```python
from build123d import *


with BuildPart() as part:
    # Esquisse1 → Révolution1 (revolve)
    with BuildSketch(Plane(origin=(0, 0, 0), x_dir=(0, 0, -1), z_dir=(1, 0, 0)), mode=Mode.PRIVATE) as r_volution1_sk:
        with BuildLine():
            Line((0, 1.5), (4, 1.5))
            Line((4, 1.5), (4, 2.15))
            Line((4, 2.15), (3, 2.15))
            ThreePointArc((3, 2.15), (3.6, 2.75), (3, 3.35))
            Line((3, 3.35), (4, 3.35))
            Line((4, 3.35), (4, 4))
            Line((4, 4), (0.903286234, 4))
            Line((0.903286234, 4), (0.903286234, 4.75))
            Line((0.903286234, 4.75), (0, 4.75))
            Line((0, 4.75), (0, 3.35))
            Line((0, 3.35), (1, 3.35))
            ThreePointArc((1, 3.35), (0.4, 2.75), (1, 2.15))
            Line((1, 2.15), (0, 2.15))
            Line((0, 2.15), (0, 1.5))
        make_face()
    revolve(r_volution1_sk.sketch.rotate(Axis((0, 0, 0), (0, 0, -1)), 90), axis=Axis((0, 0, 0), (0, 0, -1)))


solid = part.part
```
For this review, take the finished solid that the model builds, in its own axes (mm). A direction names the side the tool comes from. Give positions to 0.01 mm unless a question says otherwise; leave off trailing zeros. Write each loop counter-clockwise with the first axis right and the second up, starting at its lowest first coordinate (ties: lowest second). Pieces come first, ordered by that corner, then holes. Notation, with made-up numbers: M 60,69 L 73,69 A28 cw 73,106 Z; hole C 3.25,16 d5. An arc over 180 degrees is marked long. One line per item, written item: value.
1) Take a section at A-A, the plane y = 0. Write out the cut boundary in (x, z), then the cut area to 3 significant figures.
Results are:
outline: M -4.75,-0.9 L -4,-0.9 L -4,-4 L -3.35,-4 L -3.35,-3 A0.6 ccw -2.15,-3 L -2.15,-4 L -1.5,-4 L -1.5,0 L -2.15,0 L -2.15,-1 A0.6 ccw -3.35,-1 L -3.35,0 L -4.75,0 Z; M 1.5,-4 L 2.15,-4 L 2.15,-3 A0.6 ccw 3.35,-3 L 3.35,-4 L 4,-4 L 4,-0.9 L 4.75,-0.9 L 4.75,0 L 3.35,0 L 3.35,-1 A0.6 ccw 2.15,-1 L 2.15,0 L 1.5,0 Z
area: 18.8 mm²
2) Take a section at C-C, the plane z = -2.8. Write out the cut boundary in (x, y), then the cut area to 3 significant figures.
Results are:
outline: C 0,0 d8; hole C 0,0 d3
area: 43.2 mm²
3) The part is to be moulded in two halves that separate along X. For faces 3 (the flat face through (4, 2, -0.903)), 4 (the cylindrical face through (-2.15, -0.09, -3.49)), 5 (the cylindrical face through (-2.15, -0.09, -0.49)), 6 (the cylindrical face through (-1.03, 4.637, -0.445)), say which applies: +X half, -X half, draft (parallel to the pull), parting line (faces both ways), or undercut.
Results are:
face 3: draft
face 4: undercut
face 5: undercut
face 6: parting line
4) For P1, Ø1, axis at x = -2.5, z = -2, coming from the +Y side; P2, Ø1.5, axis at y = -2.5, z = -3.5, coming from the -X side; P3, Ø1.5, axis at x = 1.5, z = -2.5, coming from the -Y side, all flat-tipped, find the tip position at first contact; note any pin that passes through.
Results are:
P1: stops at y = 3.46
P2: stops at x = -3.6
P3: stops at y = -3.93
5) For line 1 (Y direction, x = 0, z = -3.65); line 2 (Y direction, x = -2.75, z = -3.4); line 3 (Y direction, x = 0, z = -3.4), list the stretches that pass through material, from the lowest coordinate up. Write a range as from..to.
Results are:
line 1: y = -4..-3.35, -2.15..-1.5, 1.5..2.15, 3.35..4
line 2: y = -2.9..-1.91, -1.63..1.63, 1.91..2.9
line 3: y = -4..-3.35, -3.2..-2.3, -2.15..-1.5, 1.5..2.15, 2.3..3.2, 3.35..4
6) For faces 1 (the flat face through (0.9, 1.4, 0)), 2 (the cylindrical face through (-0.867, 3.905, -2.43)), list the 3-axis set-ups (+Z, -Z, +X, -X, +Y, -Y) from which the entire face can be reached by the end or side of a thin tool; tool diameter is ignored.
Results are:
face 1: +Z, +X, -X, +Y, -Y
face 2: -Z
7) Take a section at D-D, the plane y = 3.5. Write out the cut boundary in (x, z).
Results are:
outline: M -3.21,-0.9 L -1.94,-0.9 L -1.94,-4 L 1.94,-4 L 1.94,-0.9 L 3.21,-0.9 L 3.21,0 L -3.21,0 Z
